Design review of the part shown in the three views and the two pictorial views. Dimensions are in mm from the part's minimum x, y and z. Coordinates: 2 decimals unless noted, no trailing zeros. Loops run counter-clockwise (first coordinate to the right, second up) from the corner with the lowest first, then second, coordinate; pieces in that order, holes last.
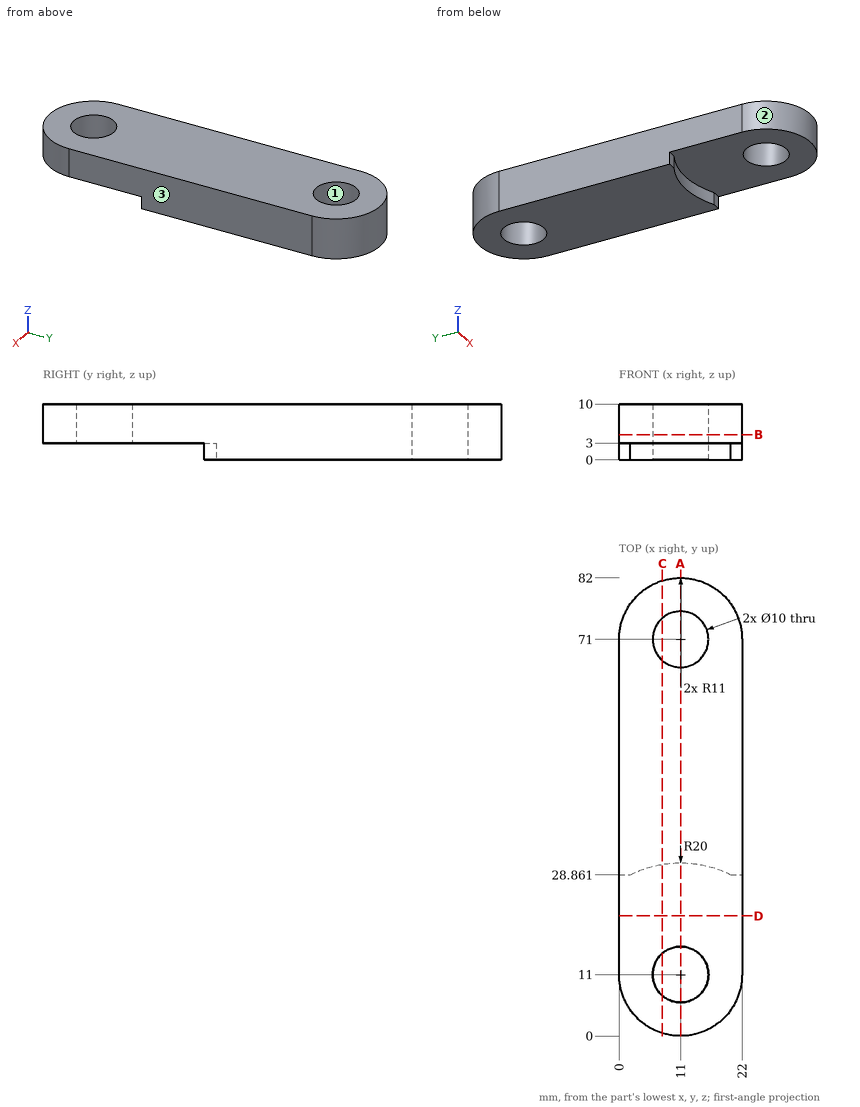
Q1. For pin 1 Ø0.6 at (x, z) = (0.5, 1) entering from -Y; pin 2 Ø6 at (x, y) = (7, 14.5) entering from -Z; pin 3 Ø1.5 at (x, z) = (12, 1.5) entering from +Y, all flat-tipped, find the tip position at first contact; note any pin that passes through.
Q2. Consider section B-B (z = 4.5). State the section outline as (x, y) points.
Q3. Wall thickness on probe 1 along Y at (x, z) = (11, 6); probe 2 along Y at (x, z) = (9.25, 6.5) (1 decimal); probe 3 along Z at (x, y) = (16, 5.5): over which ranges is each line inside the solid? List them lowest first.
Q4. Consider section C-C (x = 7.75). State the section outline as (y, z) points (1 decimal).
Q5. Consider section A-A (x = 11). State the section outline as (y, z) points, then the cut area to 3 significant figures.
Q6. The part is to be moulded in two halves that separate along X. For the marked faces 1, 2 and 3, say which applies: +X half, -X half, draft (parallel to the pull), parting line (faces both ways), or undercut.
Q7. Consider section D-D (y = 21.5). State the section outline as (x, z) points.
Model answer:
1. pin 1: stops at y = 28.86
1. pin 2: stops at z = 3
1. pin 3: stops at y = 82
2. outline: (0, 11) arc R11 ccw to (22, 11) - (22, 71) arc R11 ccw to (0, 71) - close; hole circle Ø10 at (11, 11); hole circle Ø10 at (11, 71)
3. probe 1: y = 0 to 6, 16 to 66, 76 to 82
3. probe 2: y = 0.1 to 6.3, 15.7 to 66.3, 75.7 to 81.9
3. probe 3: z = 3 to 10
4. outline: (0.5, 3) - (7.2, 3) - (7.2, 10) - (0.5, 10) - close; (14.8, 3) - (30.7, 3) - (30.7, 0) - (67.2, 0) - (67.2, 10) - (14.8, 10) - close; (74.8, 0) - (81.5, 0) - (81.5, 10) - (74.8, 10) - close
5. outline: (0, 3) - (6, 3) - (6, 10) - (0, 10) - close; (16, 3) - (31, 3) - (31, 0) - (66, 0) - (66, 10) - (16, 10) - close; (76, 0) - (82, 0) - (82, 10) - (76, 10) - close
5. area: 557 mm2
6. face 1: undercut
6. face 2: parting line
6. face 3: +X half
7. outline: (0, 3) - (22, 3) - (22, 10) - (0, 10) - close
